Design review of the part built by this model. Coordinates are the model's own, in mm. A direction names the side the tool comes from. Coordinates: 2 decimals unless noted, no trailing zeros. Loops run counter-clockwise (first coordinate to the right, second up) from the corner with the lowest first, then second, coordinate; pieces in that order, holes last. Notation, with made-up numbers: M 10.25,14 L 22.25,14 A24 ccw 22.25,24 Z; hole C 80,17 d9. An arc over 180 degrees is marked long. Put each result on its own line as item: value. Start each with the question number.
(1) The part is to be moulded in two halves that separate along Z. For faces 3 (the flat face through (-118, -209.55, 263)), 4 (the flat face through (-111, -103, 132.508)), 5 (the flat face through (-105, -107, 138.858)), say which applies: +Z half, -Z half, draft (parallel to the pull), parting line (faces both ways), or undercut.
(2) Take a section at C-C, the plane x = -100.5. Give the boundary of the cut face in (y, z).
(3) Clearance check with flat-ended pins moving along their axes: pin 1 (8 mm diameter, centred on x = -120.5, z = 227, fed in from -Y); pin 2 (2 mm diameter, centred on x = -177.5, y = -151, fed in from +Z); pin 3 (2 mm diameter, centred on x = -39.5, y = -101, fed in from +Z). State where each tip first meets the part, or that it passes through.
(4) Take a section at B-B, the plane z = 191.5. Give the boundary of the cut face in (x, y).
(5) For faces 1 (the flat face through (-126.56, -103.31, 255.13)), 2 (the flat face through (-121.09, -106.528, 251.834)), list the 3-axis set-ups (+Z, -Z, +X, -X, +Y, -Y) from which the entire face can be reached by the end or side of a thin tool; tool diameter is ignored.
(6) Take a section at A-A, the plane y = -146. Give the boundary of the cut face in (x, z).
(7) For probe 1 along Z at (x, y) = (-28.5, -154.5); probe 2 along Y at (x, z) = (-132, 232); probe 3 along X at (y, z) = (-111.5, 270), list the stretches that pass through material, from the lowest coordinate up. Write a range as [from, to].
```python
from build123d import *

# Parameters (mm, degrees)
F2_DEPTH = 6.35
F4_DEPTH = 203.2


with BuildPart() as f2:
    # F1 (on Front) → F2 (new body)
    with BuildSketch(Plane.XZ):
        Polygon((-36.510564, 374.367909), (-219.162132, 132.508471), (0, 132.508471), (0, 374.367909), align=None)
    extrude(amount=F2_DEPTH)

    # F3 (on face) → F4 (join)
    with BuildSketch(Plane.XZ.offset(6.35)):
        Polygon((-36.510564, 374.367909), (-219.162132, 132.508471), (0, 132.508471), (0, 374.367909), align=None)
        Polygon((-206.409285, 138.858471), (-33.348721, 368.017909), (-6.35, 368.017909), (-6.35, 138.858471), align=None, mode=Mode.SUBTRACT)
    extrude(amount=F4_DEPTH)


solid = f2.part
```
Computed values:
1. face 3: draft
1. face 4: -Z half
1. face 5: undercut
2. outline: M -209.55,132.51 L 0,132.51 L 0,289.64 L -209.55,289.64 L -209.55,279.1 L -6.35,279.1 L -6.35,138.86 L -209.55,138.86 Z
3. pin 1: stops at y = -6.35
3. pin 2: stops at z = 189
3. pin 3: stops at z = 371.73
4. outline: M -174.61,-209.55 L -166.65,-209.55 L -166.65,-6.35 L -6.35,-6.35 L -6.35,-209.55 L 0,-209.55 L 0,0 L -174.61,0 Z
5. face 1: +Z, -X, +Y, -Y
5. face 2: -Y
6. outline: M -219.16,132.51 L 0,132.51 L 0,374.37 L -36.51,374.37 Z; hole M -206.41,138.86 L -6.35,138.86 L -6.35,368.02 L -33.35,368.02 Z
7. probe 1: z = [132.51, 138.86], [368.02, 374.37]
7. probe 2: y = [-6.35, 0]
7. probe 3: x = [-115.33, -107.37], [-6.35, 0]
